Source: CAD feature listing. Evaluate the final solid. Frame: model axes, mm. A direction names the side the tool comes from. Give positions to 0.01 mm unless a question says otherwise; leave off trailing zeros. Loops run counter-clockwise (first coordinate to the right, second up) from the corner with the lowest first, then second, coordinate; pieces in that order, holes last. Notation, with made-up numbers: (54.5, 22.5) - (73.5, 22.5) arc R19 cw to (73.5, 37.5) - close; hole circle Ø6 at (10, 68). An arc over 180 degrees is marked (long way). Put each result on its own line as item: value.
```python
from build123d import *

# Parameters (mm, degrees)
BOSS_EXTRUDE1_DEPTH = 25.4
BOSS_EXTRUDE4_DEPTH = 25.4
SKETCH11_R          = 2.413
CUT_EXTRUDE5_DEPTH  = 10
SKETCH12_R          = 2.413
CUT_EXTRUDE6_DEPTH  = 67.32996137
CUT_EXTRUDE7_DEPTH  = 16.4


with BuildPart() as part:
    # Sketch2 → Boss-Extrude1 (new body)
    with BuildSketch(Plane.XY):
        Polygon((0, 0), (-0.197156462, 5), (-0.792344965, 10), (-1.773207125, 14.901444272), (-3.065228232, 19.490725009), (-4.786089298, 24.185257701), (-6.870037676, 28.727989265), (-9.305862968, 33.094493671), (-12.075009115, 37.252118227), (-15.162850216, 41.179727425), (-18.554323068, 44.856840338), (-22.220180921, 48.251699833), (-26.203519544, 51.392825818), (-30.362680664, 54.16796163), (-34.722984466, 56.605064941), (-39.261459458, 58.691934304), (-43.904843636, 60.400992103), (-48.717885048, 61.755478118), (-53.619641135, 62.726617227), (-63.5, 63.5), (-64.343927861, 63.5), (-64.343927861, 65.493901073), (-63.343927861, 65.493901073), (-53.346320006, 64.711340662), (-48.251922828, 63.702035375), (-43.287590163, 62.304972979), (-38.497110063, 60.541774617), (-33.81592061, 58.389282674), (-29.318144049, 55.875341756), (-25.027437614, 53.01243437), (-20.919464687, 49.773025992), (-17.137579866, 46.270716817), (-13.639271322, 42.477770187), (-10.454072963, 38.42632649), (-7.597619105, 34.137617236), (-5.085040747, 29.633523897), (-2.935391785, 24.947573759), (-1.160924955, 20.106803802), (0.172809103, 15.369357963), (1.184287688, 10.31492104), (1.798173514, 5.157850442), (1.998446984, 0.078801347), (1.920765751, -0.913615973), (0, -0.913615973), align=None)
    extrude(amount=BOSS_EXTRUDE1_DEPTH)

    # Sketch10 → Boss-Extrude4 (add, through all)
    with BuildSketch(Plane.XY.offset(25.4)):
        with BuildLine():
            Line((1.920765751, -0.913615973), (1.998446984, 0.078801347))
            Line((1.998446984, 0.078801347), (1.798173514, 5.157850442))
            Line((1.798173514, 5.157850442), (0.172809103, 15.369357963))
            Line((0.172809103, 15.369357963), (-0.873645975, 19.086384027))
            Line((-0.873645975, 19.086384027), (-3.079234249, 19.086384027))
            ThreePointArc((-3.079234249, 19.086384027), (-6.614768155, 17.621917933), (-8.079234249, 14.086384027))
            Line((-8.079234249, 14.086384027), (-8.079234249, -0.913615973))
            Line((-8.079234249, -0.913615973), (1.920765751, -0.913615973))
        make_face()
    extrude(amount=-BOSS_EXTRUDE4_DEPTH)

    # Sketch11 → Cut-Extrude5 (cut)
    with BuildSketch(Plane.XY.offset(25.4)):
        with Locations((-3.079234249, 3.086384027)):
            Circle(SKETCH11_R)
    cut_extrude5 = extrude(amount=-CUT_EXTRUDE5_DEPTH, mode=Mode.SUBTRACT)

    # Sketch12 → Cut-Extrude6 (cut, through all)
    with BuildSketch(Plane(origin=(1.998446984, 0.078801347, 0), x_dir=(0, 0, -1), z_dir=(0.999223492, 0.039400674, 0))):
        with Locations((-12.7, 7.7)):
            Circle(SKETCH12_R)
    extrude(amount=-CUT_EXTRUDE6_DEPTH, mode=Mode.SUBTRACT)

    # Mirror3: Cut-Extrude5 across plane
    add(cut_extrude5.mirror(Plane(origin=(0, 0, 12.7), x_dir=(1, 0, 0), z_dir=(0, 0, -1))), mode=Mode.SUBTRACT)

    # Sketch15 → Cut-Extrude7 (cut, through all)
    with BuildSketch(Plane(origin=(0, 0, 10), x_dir=(-1, 0, 0), z_dir=(0, 0, -1))):
        Polygon((4.48781187, 1.660586836), (4.50503144, 4.494961648), (1.670656628, 4.512181219), (1.653437058, 1.677806407), align=None)
    extrude(amount=-CUT_EXTRUDE7_DEPTH, mode=Mode.SUBTRACT)


solid = part.part
```
1) Section query B-B, the plane x = -32.5. Output: boundary loops of the cut face in (y, z), plus the area to 3 significant figures.
Check result:
outline: (55.36, 0) - (57.65, 0) - (57.65, 25.4) - (55.36, 25.4) - close
area: 58.2 mm²
2) Material intervals for line 1 along Y through (x, z) = (-6.5, 13.5); line 2 along Z through (x, y) = (-3, 8.5); line 3 along Y through (x, z) = (-38.5, 21.25), sorted ascending. Write a range as [from, to].
Check result:
line 1: [-0.91, 5.17], [9.73, 17.73], [27.92, 32.17]
line 2: [0, 10.47], [14.93, 25.4]
line 3: [58.34, 60.54]
3) Pin query (flat end, axial travel): P1, Ø3, axis at x = -3.08, y = 3.09, coming from the -Z side; P2, Ø8, axis at y = 15.5, z = 7.5, coming from the -X side; P3, Ø10, axis at y = 11.5, z = 10.5, coming from the +X side. Return the tip coordinate at first contact, or that it passes through.
Check result:
P1: z = 10
P2: x = -8.08
P3: x = 1.64
4) Access query for faces 1 (the flat face through (-3.1, 1.5, 10)), 2 (the flat face through (-3.914, 21.805, 12.522)), 3 (the flat face through (-8.079, 7, 10)), 4 (the cylindrical face through (-3.39, 5.48, 20.47)). Directions: +Z, -Z, +X, -X, +Y, -Y. A direction counts if a zero-diameter tool reaches every point of the face in a straight line with its end or side. Return the directions, or none.
Check result:
face 1: -Z
face 2: +Z, -Z, -X
face 3: +Z, -Z, -X, -Y
face 4: +Z
5) Mould query, pull axis Z, two halves, no side actions, for faces 5 (the flat face through (-58.491, 63.108, 12.522)), 6 (the cylindrical face through (-3.13, 6.66, 10.47)), 7 (the flat face through (-3.1, 1.5, 15.4)). Classes: pulls with the +Z half, pulls with the -Z half, needs draft (parallel to the pull), parting line crosses it, or undercut.
Check result:
face 5: needs draft
face 6: undercut
face 7: pulls with the +Z half
6) Section query A-A, the plane y = 26.5. Output: boundary loops of the cut face in (x, z), plus the area to 3 significant figures.
Check result:
outline: (-5.85, 0) - (-3.65, 0) - (-3.65, 25.4) - (-5.85, 25.4) - close
area: 55.9 mm²
